The model under review builds one solid part; all positions refer to its coordinate system, in mm. A direction names the side the tool comes from. Round coordinates to 2 decimals unless told otherwise and drop trailing zeros. Order: outer loops, then holes, each group sorted by start corner. A loop starts at its lowest first (then second) coordinate and runs counter-clockwise, first axis right, second up. Notation, with made-up numbers: M 45,51.25 L 61,51.25 A18 ccw 61,83.25 Z; hole C 62,35.5 d3. An arc over 180 degrees is marked long. One line per item, written item: value. Start each with the question number.
from build123d import *

# Parameters (mm, degrees)
P_IDAT_VYSUNUT_M1_DEPTH                           = 46.5
P_IDAT_VYSUNUT_M2_DEPTH                           = 6.5
V_LCOV_ZAHLOUBEN_PRO_M6_ROUBY_S_V_LCO_D           = 6.6
V_LCOV_ZAHLOUBEN_PRO_M6_ROUBY_S_V_LCO_CBORE_D     = 13
V_LCOV_ZAHLOUBEN_PRO_M6_ROUBY_S_V_LCO_CBORE_DEPTH = 4.6
SKICA6_R                                          = 5
ODEBRAT_VYSUNUT_M1_DEPTH                          = 93.485133941
SKICA7_W                                          = 73
SKICA7_H                                          = 28
ODEBRAT_VYSUNUT_M2_DEPTH                          = 2
ODEBRAT_START                                     = -10
SKICA8_W                                          = 97
SKICA8_H                                          = 52
SKICA8_W_2                                        = 77
SKICA8_H_2                                        = 32
ODEBRAT_VYSUNUT_M5_DEPTH                          = 10
SKICA9_W                                          = 6
SKICA9_H                                          = 5
P_IDAT_VYSUNUT_M3_DEPTH                           = 2
D_RY_PRO_KOL_K_VELIKOST_MM1_REACH                 = 76.356
D_RY_PRO_KOL_K_VELIKOST_MM1_BORE_R                = 1.95


with BuildPart() as part:
    # Skica1 → P_idat vysunut_m1 (new body)
    with BuildSketch(Plane.XY):
        with BuildLine():
            Line((-32.5, -21.5), (0, -21.5))
            Line((0, -21.5), (32.5, -21.5))
            ThreePointArc((32.5, -21.5), (39.571067812, -18.571067812), (42.5, -11.5))
            Line((42.5, -11.5), (42.5, 11.5))
            ThreePointArc((42.5, 11.5), (39.571067812, 18.571067812), (32.5, 21.5))
            Line((32.5, 21.5), (-32.5, 21.5))
            ThreePointArc((-32.5, 21.5), (-39.571067812, 18.571067812), (-42.5, 11.5))
            Line((-42.5, 11.5), (-42.5, -11.5))
            ThreePointArc((-42.5, -11.5), (-39.571067812, -18.571067812), (-32.5, -21.5))
        make_face()
        Polygon((-34.5, -8.5), (-34.5, 13.5), (34.5, 13.5), (34.5, -8.5), (36.5, -8.5), (36.5, -10.5), (34.5, -10.5), (34.5, -13.5), (0, -13.5), (-34.5, -13.5), (-34.5, -10.5), (-36.5, -10.5), (-36.5, -8.5), align=None, mode=Mode.SUBTRACT)
    extrude(amount=P_IDAT_VYSUNUT_M1_DEPTH)

    # Skica2 → P_idat vysunut_m2 (add)
    with BuildSketch(Plane(origin=(0, 0, 0), x_dir=(-1, 0, 0), z_dir=(0, 0, -1))):
        Polygon((34.5, 11.5), (-34.5, 11.5), (-34.5, -8.5), (-36.5, -8.5), (-36.5, -10.5), (-34.5, -10.5), (-34.5, -11.5), (34.5, -11.5), (34.5, -10.5), (36.5, -10.5), (36.5, -8.5), (34.5, -8.5), align=None)
        Polygon((-10, 7.5), (10, 7.5), (10, -7.5), (-10, -7.5), (-10, 0), align=None, mode=Mode.SUBTRACT)
    extrude(amount=-P_IDAT_VYSUNUT_M2_DEPTH)

    # V_lcov_ zahlouben_ pro M6 _rouby s v_lco (through all)
    with Locations(Plane.XY.offset(6.5)):
        with Locations((-19, 0), (19, 0)):
            CounterBoreHole(V_LCOV_ZAHLOUBEN_PRO_M6_ROUBY_S_V_LCO_D / 2, V_LCOV_ZAHLOUBEN_PRO_M6_ROUBY_S_V_LCO_CBORE_D / 2, V_LCOV_ZAHLOUBEN_PRO_M6_ROUBY_S_V_LCO_CBORE_DEPTH)

    # Skica6 → Odebrat vysunut_m1 (cut, through all)
    with BuildSketch(Plane.ZY.offset(-34.5)):
        with Locations((11.5, 2.5)):
            Circle(SKICA6_R)
    extrude(amount=-ODEBRAT_VYSUNUT_M1_DEPTH, mode=Mode.SUBTRACT)

    # Skica7 → Odebrat vysunut_m2 (cut)
    with BuildSketch(Plane.XY.offset(46.5)):
        Rectangle(SKICA7_W, SKICA7_H)
    extrude(amount=-ODEBRAT_VYSUNUT_M2_DEPTH, mode=Mode.SUBTRACT)

    # Skica8 → Odebrat vysunut_m5 (cut)
    # profile 1 of 2: a face of its own
    with BuildSketch(Plane.XY.offset(46.5).offset(ODEBRAT_START)):
        Rectangle(SKICA8_W, SKICA8_H)
        with BuildLine():
            Line((-32.5, -21.5), (32.5, -21.5))
            ThreePointArc((32.5, -21.5), (39.571067812, -18.571067812), (42.5, -11.5))
            Line((42.5, -11.5), (42.5, 11.5))
            ThreePointArc((42.5, 11.5), (39.571067812, 18.571067812), (32.5, 21.5))
            Line((32.5, 21.5), (-32.5, 21.5))
            ThreePointArc((-32.5, 21.5), (-39.571067812, 18.571067812), (-42.5, 11.5))
            Line((-42.5, 11.5), (-42.5, -11.5))
            ThreePointArc((-42.5, -11.5), (-39.571067812, -18.571067812), (-32.5, -21.5))
        make_face(mode=Mode.SUBTRACT)
    # profile 2 of 2: a face of its own
    with BuildSketch(Plane.XY.offset(46.5).offset(ODEBRAT_START)):
        with BuildLine():
            ThreePointArc((-42.5, -11.5), (-39.571067812, -18.571067812), (-32.5, -21.5))
            Line((-32.5, -21.5), (32.5, -21.5))
            ThreePointArc((32.5, -21.5), (39.571067812, -18.571067812), (42.5, -11.5))
            Line((42.5, -11.5), (42.5, 11.5))
            ThreePointArc((42.5, 11.5), (39.571067812, 18.571067812), (32.5, 21.5))
            Line((32.5, 21.5), (-32.5, 21.5))
            ThreePointArc((-32.5, 21.5), (-39.571067812, 18.571067812), (-42.5, 11.5))
            Line((-42.5, 11.5), (-42.5, -11.5))
        make_face()
        Rectangle(SKICA8_W_2, SKICA8_H_2, mode=Mode.SUBTRACT)
    extrude(amount=ODEBRAT_VYSUNUT_M5_DEPTH, mode=Mode.SUBTRACT)

    # Skica9 → P_idat vysunut_m3 (add)
    with BuildSketch(Plane(origin=(0, 16, 0), x_dir=(1, 0, 0), z_dir=(0, 1, 0))):
        with Locations((-23, -44)):
            Rectangle(SKICA9_W, SKICA9_H)
        with Locations((-23, -39)):
            Rectangle(SKICA9_W, SKICA9_H)
        with Locations((23, -44)):
            Rectangle(SKICA9_W, SKICA9_H)
        with Locations((23, -39)):
            Rectangle(SKICA9_W, SKICA9_H)
    p_idat_vysunut_m3 = extrude(amount=P_IDAT_VYSUNUT_M3_DEPTH)

    # Zrcadlit1: P_idat vysunut_m3 across plane
    add(p_idat_vysunut_m3.mirror(Plane(origin=(0, 0, 0), x_dir=(0, 0, 1), z_dir=(0, -1, 0))))

    # D_ry pro kol_k_ velikost mm1 bore → D_ry pro kol_k_ velikost mm1 (cut, up to next)
    with BuildSketch(Plane(origin=(0, -18, 0), x_dir=(-1, 0, 0), z_dir=(0, -1, 0)), mode=Mode.PRIVATE) as d_ry_pro_kol_k_velikost_mm1_sk1:
        with Locations((-23, -41.5)):
            Circle(D_RY_PRO_KOL_K_VELIKOST_MM1_BORE_R)
    d_ry_pro_kol_k_velikost_mm1_tool1 = extrude(d_ry_pro_kol_k_velikost_mm1_sk1.sketch, amount=-D_RY_PRO_KOL_K_VELIKOST_MM1_REACH, mode=Mode.PRIVATE) & part.part
    # D_ry pro kol_k_ velikost mm1 bore → D_ry pro kol_k_ velikost mm1 (cut, up to next)
    with BuildSketch(Plane(origin=(0, -18, 0), x_dir=(-1, 0, 0), z_dir=(0, -1, 0)), mode=Mode.PRIVATE) as d_ry_pro_kol_k_velikost_mm1_sk2:
        with Locations((23, -41.5)):
            Circle(D_RY_PRO_KOL_K_VELIKOST_MM1_BORE_R)
    d_ry_pro_kol_k_velikost_mm1_tool2 = extrude(d_ry_pro_kol_k_velikost_mm1_sk2.sketch, amount=-D_RY_PRO_KOL_K_VELIKOST_MM1_REACH, mode=Mode.PRIVATE) & part.part
    d_ry_pro_kol_k_velikost_mm1_1 = d_ry_pro_kol_k_velikost_mm1_tool1.solids().sort_by_distance((23, -18, 41.5))[0]
    add(d_ry_pro_kol_k_velikost_mm1_1, mode=Mode.SUBTRACT)
    d_ry_pro_kol_k_velikost_mm1_2 = d_ry_pro_kol_k_velikost_mm1_tool2.solids().sort_by_distance((-23, -18, 41.5))[0]
    add(d_ry_pro_kol_k_velikost_mm1_2, mode=Mode.SUBTRACT)
    d_ry_pro_kol_k_velikost_mm1 = d_ry_pro_kol_k_velikost_mm1_1 + d_ry_pro_kol_k_velikost_mm1_2  # D_ry pro kol_k_ velikost mm1 as one shape, for the pattern or mirror that repeats it

    # Zrcadlit2: D_ry pro kol_k_ velikost mm1 across plane
    add(d_ry_pro_kol_k_velikost_mm1.mirror(Plane(origin=(0, 0, 0), x_dir=(0, 0, 1), z_dir=(0, -1, 0))), mode=Mode.SUBTRACT)


solid = part.part
Item 1: Wall thickness on L1, parallel to X at y = 15.35, z = 41.5; L2, parallel to Y at x = -9.5, z = 33; L3, parallel to Y at x = -19, z = 0.95: over which ranges is each line inside the solid? List them lowest first.
Item 2: Consider section B-B, the plane y = 9. Give the boundary of the cut face in (x, z).
Item 3: Consider section C-C, the plane z = 24. Give the boundary of the cut face in (x, y).
Item 4: The part is to be moulded in two halves that separate along X. For faces 1 (the flat face through (26, -17, 42)), 2 (the flat face through (0, -7.5, 3)), 3 (the flat face through (32, -16, 41)), say which applies: pulls with the +X half, pulls with the -X half, needs draft (parallel to the pull), parting line crosses it, or undercut.
Item 5: Consider section A-A, the plane x = 19. Give the boundary of the cut face in (y, z), then the cut area to 3 significant figures.
Item 6: Machinability: for faces 4 (the flat face through (23, -18, 39)), 5 (the flat face through (-32, 16, 41)), 6 (the flat face through (23, 18, 39)), which of the approach directions +Z, -Z, +X, -X, +Y, -Y give a long, thin tool a straight path to every point of the face, cutting with its end or side? Answer none if there is none.
Item 7: Clearance check with flat-ended pins moving along their axes: P1, Ø4.5, axis at x = 23, z = 41.5, coming from the -Y side; P2, Ø5, axis at y = 4.5, z = 44, coming from the -X side; P3, Ø1.5, axis at x = -13, z = 38.5, coming from the -Y side. State where each tip first meets the part, or that it passes through.
Item 8: Consider section D-D, the plane y = -4.5. Give the boundary of the cut face in (x, z), then the cut area to 3 significant figures.
Computed:
1. L1: x = -38.5 to -24.95, -21.05 to 21.05, 24.95 to 38.5
1. L2: y = -21.5 to -13.5, 13.5 to 21.5
1. L3: y = -21.5 to -13.5, -11.5 to -3.3, 3.3 to 11.5, 13.5 to 21.5
2. outline: M -42.5,0 L 42.5,0 L 42.5,36.5 L 38.5,36.5 L 38.5,46.5 L 36.5,46.5 L 36.5,44.5 L 34.5,44.5 L 34.5,6.5 L -34.5,6.5 L -34.5,44.5 L -36.5,44.5 L -36.5,46.5 L -38.5,46.5 L -38.5,36.5 L -42.5,36.5 Z
3. outline: M -42.5,-11.5 A10 ccw -32.5,-21.5 L 32.5,-21.5 A10 ccw 42.5,-11.5 L 42.5,11.5 A10 ccw 32.5,21.5 L -32.5,21.5 A10 ccw -42.5,11.5 Z; hole M -36.5,-10.5 L -34.5,-10.5 L -34.5,-13.5 L 34.5,-13.5 L 34.5,-10.5 L 36.5,-10.5 L 36.5,-8.5 L 34.5,-8.5 L 34.5,13.5 L -34.5,13.5 L -34.5,-8.5 L -36.5,-8.5 Z
4. face 1: pulls with the +X half
4. face 2: undercut
4. face 3: needs draft
5. outline: M -21.5,0 L -13.5,0 L -13.5,44.5 L -14,44.5 L -14,46.5 L -16,46.5 L -16,36.5 L -21.5,36.5 Z; M -11.5,0 L -3.3,0 L -3.3,1.9 L -6.5,1.9 L -6.5,6.5 L -11.5,6.5 Z; M 3.3,0 L 11.5,0 L 11.5,6.5 L 6.5,6.5 L 6.5,1.9 L 3.3,1.9 Z; M 13.5,0 L 21.5,0 L 21.5,36.5 L 16,36.5 L 16,46.5 L 14,46.5 L 14,44.5 L 13.5,44.5 Z
5. area: 709 mm^2
6. face 4: +Z, +X, -X, -Y
6. face 5: +Z, -X, +Y
6. face 6: +Z, +X, -X, +Y
7. P1: stops at y = -18
7. P2: stops at x = -38.5
7. P3: stops at y = -16
8. outline: M -42.5,0 L -10,0 L -10,6.5 L -14.31,6.5 L -14.31,1.9 L -23.69,1.9 L -23.69,6.5 L -34.5,6.5 L -34.5,44.5 L -36.5,44.5 L -36.5,46.5 L -38.5,46.5 L -38.5,36.5 L -42.5,36.5 Z; M 10,0 L 42.5,0 L 42.5,36.5 L 38.5,36.5 L 38.5,46.5 L 36.5,46.5 L 36.5,44.5 L 34.5,44.5 L 34.5,6.5 L 23.69,6.5 L 23.69,1.9 L 14.31,1.9 L 14.31,6.5 L 10,6.5 Z
8. area: 888 mm^2
